Geometry: final body of the model. Coordinates: model frame, mm. Give positions to 0.01 mm unless a question says otherwise; leave off trailing zeros. Loops run counter-clockwise (first coordinate to the right, second up) from the corner with the lowest first, then second, coordinate; pieces in that order, holes last. Notation, with made-up numbers: (-5, 68.25) - (8, 68.25) arc R22 cw to (8, 76.25) - close; hole circle Ø9 at (60, 58.25). An arc over 180 degrees is marked (long way). Use one line per item in the form item = value.
```python
from build123d import *

# Parameters (mm, degrees)
SKETCH1_W                  = 10
SKETCH1_H                  = 100
BOSS_EXTRUDE1_DEPTH        = 6
F_2_5_2_5_DIAMETER_HOLE1_D = 2.5
F_2_5_2_5_DIAMETER_HOLE2_D = 2.5


with BuildPart() as part:
    # Sketch1 → Boss-Extrude1 (new body)
    with BuildSketch(Plane.XY.offset(6)):
        Rectangle(SKETCH1_W, SKETCH1_H)
    extrude(amount=-BOSS_EXTRUDE1_DEPTH)

    # Ø2.5 (2.5) Diameter Hole1 (through all)
    with Locations(Plane.XY.offset(6)):
        with Locations((0, 45), (0, -45)):
            Hole(F_2_5_2_5_DIAMETER_HOLE1_D / 2)

    # Ø2.5 (2.5) Diameter Hole2 (through all)
    with Locations(Plane(origin=(5, 0, 0), x_dir=(0, 0, -1), z_dir=(1, 0, 0))):
        with Locations((-3, 40), (-3, -40)):
            Hole(F_2_5_2_5_DIAMETER_HOLE2_D / 2)


solid = part.part
```
(1) Material intervals for L1, parallel to Y at x = 0, z = 1.3; L2, parallel to Y at x = -2, z = 3; L3, parallel to Y at x = 0, z = 3.4, sorted ascending. Write a range as from..to.
Solution:
L1 = -50..-46.25, -43.75..43.75, 46.25..50
L2 = -50..-41.25, -38.75..38.75, 41.25..50
L3 = -50..-46.25, -43.75..-41.18, -38.82..38.82, 41.18..43.75, 46.25..50
(2) Cut plane A-A (z = 3). Return the cut outline in (x, y), plus the area to 3 significant figures.
Solution:
outline = (-5, -50) - (5, -50) - (5, -41.25) - (-5, -41.25) - close; (-5, -38.75) - (5, -38.75) - (5, 38.75) - (-5, 38.75) - close; (-5, 41.25) - (5, 41.25) - (5, 50) - (-5, 50) - close; hole circle Ø2.5 at (0, -45); hole circle Ø2.5 at (0, 45)
area = 940 mm2
(3) Cut plane C-C (y = -40). Return the cut outline in (x, z).
Solution:
outline = (-5, 0) - (5, 0) - (5, 1.75) - (-5, 1.75) - close; (-5, 4.25) - (5, 4.25) - (5, 6) - (-5, 6) - close
(4) Pull-direction query (Z, two-part tool) for faces 1 (the face through (-0.07, -41.109, 3.577)), 2 (the face through (5, -1, 3)), 3 (the face through (0, 1, 6)); classes: released by +Z, released by -Z, zero draft, split by the parting line, or undercut.
Solution:
face_1 = undercut
face_2 = zero draft
face_3 = released by +Z
(5) Pin query (flat end, axial travel): P1, Ø2, axis at x = 0, y = 45, coming from the +Z side. Return the tip coordinate at first contact, or that it passes through.
Solution:
P1 = through
(6) Cut plane B-B (x = 0). Return the cut outline in (y, z).
Solution:
outline = (-50, 0) - (-46.25, 0) - (-46.25, 6) - (-50, 6) - close; (-43.75, 0) - (43.75, 0) - (43.75, 6) - (-43.75, 6) - close; (46.25, 0) - (50, 0) - (50, 6) - (46.25, 6) - close; hole circle Ø2.5 at (-40, 3); hole circle Ø2.5 at (40, 3)
